Verification items for the finished model (mm, model axes). A direction names the side the tool comes from. Round coordinates to 2 decimals unless told otherwise and drop trailing zeros. Write each loop counter-clockwise with the first axis right and the second up, starting at its lowest first coordinate (ties: lowest second). Pieces come first, ordered by that corner, then holes. Notation, with made-up numbers: (-6.75, 15) - (47.25, 15) arc R22 ccw to (47.25, 26) - close; hole circle Ø10 at (25.25, -5). An arc over 180 degrees is marked (long way). Answer as a JSON object with one key per item and string values. Group by question number.
1) Thickness scan on line 1 (Y direction, x = 0, z = -82.4); line 2 (Y direction, x = -16, z = -82.25); line 3 (X direction, y = 0, z = -81.15). Record the ranges inside material, lowest first.
2) Mould release check, pull along Y, two halves, no side actions. Record for faces 3 (the flat face through (-8.7, -4.3, -83)), 4 (the cylindrical face through (-16.45, 0.05, -81.73)), 5 (the cylindrical face through (5.448, -0.163, -82.958)): +Y half, -Y half, draft (parallel to the pull), parting line (faces both ways), or undercut.
3) Set-up check for faces 1 (the flat face through (-8.187, 2.724, -81.726)), 2 (the cylindrical face through (0.54, -2.44, -84.73)): record each of +Z, -Z, +X, -X, +Y, -Y from which the full face is reachable in a straight line by a thin tool's end or side.
4) Go/stop test with flat-tipped pins: pin 1 Ø7 at (x, y) = (0, 0) entering from -Z; pin 2 Ø1 at (y, z) = (-27.5, -84.5) entering from -X; pin 3 Ø2 at (x, z) = (-29, -81) entering from +Y; pin 4 Ø1.5 at (x, z) = (-20.5, -84) entering from +Y. Record where each tip stops, or that it passes through.
5) Section check B-B (x = -6). Enter the section's corners in (y, z).
6) Section check A-A (x = 0). Enter the section's corners in (y, z), then the cut area to 4 significant figures.
```python
from build123d import *

# Parameters (mm, degrees)
BOSS_EXTRUDE1_DEPTH = 6
CUT_EXTRUDE1_DEPTH  = 3.5
SKETCH4_R           = 2.5
CUT_EXTRUDE2_DEPTH  = 3.5
SKETCH6_RX          = 2.368753343
SKETCH6_RY          = 2.322011883
CUT_EXTRUDE3_DEPTH  = 30


with BuildPart() as part:
    # Sketch1 → Boss-Extrude1 (new body)
    with BuildSketch(Plane.XY):
        with BuildLine():
            Line((-14.268243934, -3.994041761), (-2.898518265, -4.615310593))
            ThreePointArc((-2.898518265, -4.615310593), (5.45, 0), (-2.898518265, 4.615310593))
            Line((-2.898518265, 4.615310593), (-14.17529192, 4.292464798))
            add(Edge.make_bspline(
                [(-14.17529192, 4.292464798), (-42.462260129, 4.288818218), (-52.533757866, -18.372051692), (-36.302785322, -42.655354232)],
                knots=[0, 0, 0, 0, 1, 1, 1, 1], degree=3))
            ThreePointArc((-36.302785322, -42.655354232), (-33.552833422, -43.610103827), (-32.640753317, -40.845706583))
            add(Edge.make_bspline(
                [(-14.268243934, -3.994041761), (-34.73116579, -2.87481632), (-47.018413867, -18.971545605), (-32.640753317, -40.845706583)],
                knots=[0, 0, 0, 0, 1, 1, 1, 1], degree=3))
        make_face()
    extrude(amount=BOSS_EXTRUDE1_DEPTH)

    # Sketch3 → Cut-Extrude1 (cut)
    with BuildSketch(Plane.XY):
        with BuildLine():
            Line((-14.18094636, -2.396425056), (-2.359318085, -3.042386921))
            ThreePointArc((-2.359318085, -3.042386921), (3.85, 0), (-2.359318085, 3.042386921))
            Line((-2.359318085, 3.042386921), (-14.18094636, 2.396425056))
            ThreePointArc((-14.18094636, 2.396425056), (-16.45, 0), (-14.18094636, -2.396425056))
        make_face()
    extrude(amount=CUT_EXTRUDE1_DEPTH, mode=Mode.SUBTRACT)

    # Sketch4 → Cut-Extrude2 (cut)
    with BuildSketch(Plane(origin=(0, 0, 3.5), x_dir=(-1, 0, 0), z_dir=(0, 0, -1))):
        Circle(SKETCH4_R)
    extrude(amount=-CUT_EXTRUDE2_DEPTH, mode=Mode.SUBTRACT)

    # Sketch6 → Cut-Extrude3 (cut)
    with BuildSketch(Plane(origin=(-23.619287881, -25.215704234, 0), x_dir=(0, 0, -1), z_dir=(0.683626277, 0.72983225, 0))):
        with Locations(Location((-3, -5.45537074), (0, 0, -90))):
            Ellipse(SKETCH6_RX, SKETCH6_RY)
    extrude(amount=-CUT_EXTRUDE3_DEPTH, mode=Mode.SUBTRACT)


with BuildPart() as body_2:
    # Mirror3: mirrored copy
    add(part.part.mirror(Plane(origin=(0, 0, -40), x_dir=(1, 0, 0), z_dir=(0, 0, -1))))


solid = body_2.part
```
Returned:
{
 "1": {"line 1": "-5.45 to -3.85, 3.85 to 5.45", "line 2": "-3.94 to -1.4, 1.4 to 4.26", "line 3": "-32.52 to -16.45, 3.85 to 5.45"},
 "2": {"face 3": "-Y half", "face 4": "undercut", "face 5": "parting line"},
 "3": {"face 1": "+Z", "face 2": "+Z, -Z"},
 "4": {"pin 1": "z = -86", "pin 2": "x = -43.3", "pin 3": "y = 2.08", "pin 4": "y = 3.98"},
 "5": {"outline": "(-4.45, -86) - (4.53, -86) - (4.53, -80) - (2.84, -80) - (2.84, -83.5) - (-2.84, -83.5) - (-2.84, -80) - (-4.45, -80) - close"},
 "6": {"outline": "(-5.45, -86) - (-2.5, -86) - (-2.5, -83.5) - (-3.85, -83.5) - (-3.85, -80) - (-5.45, -80) - close; (2.5, -86) - (5.45, -86) - (5.45, -80) - (3.85, -80) - (3.85, -83.5) - (2.5, -83.5) - close", "area": "25.95 mm2"}
}
